from build123d import *

# Parameters (mm, degrees)
SKETCH_1_R      = 5
EXTRUDE_1_DEPTH = 70
SKETCH_2_R      = 5
EXTRUDE_2_DEPTH = 50
SKETCH_3_R      = 15
EXTRUDE_3_DEPTH = 20
SKETCH_4_R      = 5
EXTRUDE_4_DEPTH = 90
SKETCH_8_R      = 5
EXTRUDE_5_DEPTH = 90
SKETCH_9_R      = 5
EXTRUDE_6_DEPTH = 90


with BuildPart() as part:
    # Sketch 1 → Extrude 1 (new body, symmetric)
    with BuildSketch(Plane.XY):
        Circle(SKETCH_1_R)
    extrude(amount=EXTRUDE_1_DEPTH, both=True)

    # Sketch 2 → Extrude 2 (add)
    with BuildSketch(Plane(origin=(0, 0, -70), x_dir=(-1, 0, 0), z_dir=(0, 0, -1))):
        Circle(SKETCH_2_R)
    extrude(amount=EXTRUDE_2_DEPTH)

    # Sketch 3 → Extrude 3 (add)
    with BuildSketch(Plane(origin=(0, 0, -120), x_dir=(-1, 0, 0), z_dir=(0, 0, -1))):
        Circle(SKETCH_3_R)
    extrude(amount=EXTRUDE_3_DEPTH)

    # Sketch 4 → Extrude 4 (add)
    with BuildSketch(Plane(origin=(0, 0, 0), x_dir=(1, 0, 0), z_dir=(0, 1, 0))):
        with Locations((0, 130)):
            Circle(SKETCH_4_R)
    extrude(amount=EXTRUDE_4_DEPTH)

    # Sketch 8 → Extrude 5 (add)
    with BuildSketch(Plane(origin=(0, 0, 0), x_dir=(0, 0, -1), z_dir=(0.866025404, -0.5, 0))):
        with Locations((130, 0)):
            Circle(SKETCH_8_R)
    extrude(amount=EXTRUDE_5_DEPTH)

    # Sketch 9 → Extrude 6 (add)
    with BuildSketch(Plane(origin=(0, 0, 0), x_dir=(0, 0, 1), z_dir=(-0.866025404, -0.5, 0))):
        with Locations((-130, 0)):
            Circle(SKETCH_9_R)
    extrude(amount=EXTRUDE_6_DEPTH)


solid = part.part
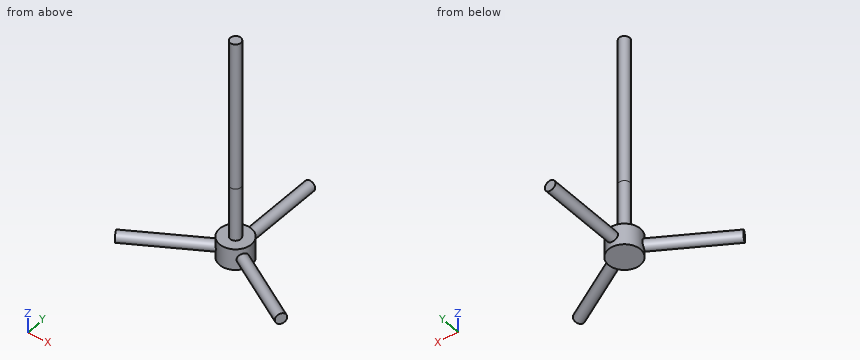
The listing builds one solid part. Answer for the finished solid, in the listing's coordinates (mm). Give positions to 0.01 mm unless a question says otherwise; leave off trailing zeros. Order: outer loops, then holes, each group sorted by start corner. A loop starts at its lowest first (then second) coordinate and runs counter-clockwise, first axis right, second up. Notation, with made-up numbers: (2.5, 47) - (21.5, 47) arc R14 ccw to (21.5, 67) - close; hole circle Ø6 at (-24.5, 42.5). An arc over 180 degrees is marked (long way). Use one line per item in the form item = value.
1) Each of these flat-tipped pins is pushed along its axis until it touches: pin 1 (1.5 mm diameter, centred on x = 41.5, y = -28, fed in from -Z); pin 2 (12 mm diameter, centred on x = -24, y = 8, fed in from -Z). Where does it stop, or does it pass through?
Verdict:
pin_1 = -134.18
pin_2 = through
2) Find section D-D on y = 44.5. Determine the outline of the cut face in (x, z).
Verdict:
outline = circle Ø10 at (0, -130)
3) Find section B-B on y = 0. Determine the outline of the cut face in (x, z), and give its area (3 significant figures).
Verdict:
outline = (-15, -140) - (15, -140) - (15, -120) - (5, -120) - (5, 70) - (-5, 70) - (-5, -120) - (-15, -120) - close
area = 2,500 mm^2
4) Consider probe 1 along X at (y, z) = (58.5, -129.5); probe 2 along Z at (x, y) = (56.5, -32); probe 3 along Y at (x, z) = (2, 42.5). Determine where each line is inside the solid, lowest interval first. Write a range as [from, to].
Verdict:
probe_1 = [-4.97, 4.97]
probe_2 = [-134.97, -125.03]
probe_3 = [-4.58, 4.58]
5) Find section C-C on z = -33.5. Determine the outline of the cut face in (x, y).
Verdict:
outline = circle Ø10 at (0, 0)
6) Find section A-A on x = 0. Determine the outline of the cut face in (y, z).
Verdict:
outline = (-15, -140) - (15, -140) - (15, -135) - (90, -135) - (90, -125) - (15, -125) - (15, -120) - (5, -120) - (5, 70) - (-5, 70) - (-5, -120) - (-15, -120) - close
